Autodesk Inventor part; units mm, degrees
ref_plane "YZ Plane" through (0, 0, 0) normal (1, 0, 0) x (0, 1, 0)
ref_plane "XZ Plane" through (0, 0, 0) normal (0, 1, 0) x (-1, 0, 0)
ref_plane "XY Plane" through (0, 0, 0) normal (0, 0, 1) x (1, 0, 0)
sketch "Sketch1" plane through (0, 0, 0) normal (0, 1, 0) x (-1, 0, 0)
  arc A0 (-99.8914, -75.1446) -> (-99.8914, 75.1446) centre (0, 0) ccw
  line L0 (-65, 0) -> (-65, 55)
  line L1 (-65, 55) -> (-99.8914, 75.1446)
  line L2 (-65, 0) -> (-65, -55)
  line L3 (-65, -55) -> (-99.8914, -75.1446)
  dimension "d0" = 250
  dimension "d4" = 55
  dimension "d6" = 120
extrude "Extrusion1" add sketch "Sketch1" along normal blind 5
sketch "Sketch2" plane through (0, 5, 0) normal (0, 1, 0) x (1, 0, 0)
  line L0 (-70, 15) -> (15, 15)
  line L1 (15, 40) -> (-70, 40)
  arc A0 (15, 15) -> (15, 40) centre (15, 27.5) ccw
  arc A1 (-70, 40) -> (-70, 15) centre (-70, 27.5) ccw
  line L2 (65, -55) -> (65, 55)
  line L3 (-70, -15) -> (15, -15)
  line L4 (15, -40) -> (-70, -40)
  arc A2 (15, -40) -> (15, -15) centre (15, -27.5) ccw
  arc A3 (-70, -15) -> (-70, -40) centre (-70, -27.5) ccw
  point P0 (0, 0)
extrude "Extrusion2" cut sketch "Sketch2" against normal blind 10
sketch "Sketch3" plane through (0, 5, 0) normal (0, 1, 0) x (1, 0, 0)
  circle A0 centre (-105, 0) radius 4
  circle A1 centre (0, 105) radius 4.3333
  circle A2 centre (0, -105) radius 4.3461
  arc A3 (99.8914, 75.1446) -> (99.8914, -75.1446) centre (0, 0) ccw
  dimension "d25" = 8
  dimension "d26" = 105
  dimension "d27" = 105
  dimension "d28" = 105
extrude "Extrusion3" cut sketch "Sketch3" against normal blind 10
sketch "Sketch4" plane through (0, 5, 0) normal (0, 1, 0) x (1, 0, 0)
  circle A0 centre (-59.9853, -55) radius 2.5
  circle A1 centre (-29.9853, -55) radius 5
  circle A2 centre (0.0147, -55) radius 5
  line L0 (-104.2134, 0) -> (86.9491, 0)
  point P0 (0, 0)
  dimension "d31" = 5
  dimension "d32" = 10
  dimension "d33" = 10
  dimension "d34" = 55
  dimension "d35" = 55
  dimension "d36" = 55
  dimension "d37" = 30
  dimension "d38" = 30
extrude "Extrusion4" add sketch "Sketch4" along normal blind 10
fillet "Fillet2" radius 2 1 edges at (-62.4853, 15, 55)
chamfer "Chamfer1" distance 1.25 angle 45 1 edges at (-4.9853, 15, 55)
chamfer "Chamfer2" distance 1.25 angle 45 1 edges at (-34.9853, 15, 55)
sketch "Sketch5" plane through (0, 5, 0) normal (0, 1, 0) x (1, 0, 0)
  line L0 (-35.937, -60.9099) -> (-23.937, -60.9099)
  line L1 (-23.937, -60.9099) -> (-23.937, -48.9099)
  line L2 (-23.937, -48.9099) -> (-35.937, -48.9099)
  line L3 (-35.937, -48.9099) -> (-35.937, -60.9099)
  point P0 (0, 0)
  point P1 (-29.437, -54.7059)
  point P2 (-29.437, -54.7059)
  dimension "d50" = 12
  dimension "d51" = 12
  dimension "d52" = 6.5
  dimension "d53" = 5.796
extrude "Extrusion5" add sketch "Sketch5" along normal blind 0.05
sketch "Sketch6" plane through (0, 5, 0) normal (0, 1, 0) x (1, 0, 0)
  line L0 (-36.7143, -61.9407) -> (-23.1511, -61.9407) construction
  line L1 (-23.1511, -61.9407) -> (-23.1511, -65.2373) construction
  line L2 (-23.1511, -65.2373) -> (-36.7143, -65.2373) construction
  line L3 (-36.7143, -65.2373) -> (-36.7143, -61.9407) construction
  point P0 (0, 0)
properties part number "Top and middle round"
Design review of the part built by this model. Coordinates are the model's own, in mm. A direction names the side the tool comes from. Round coordinates to 2 decimals unless told otherwise and drop trailing zeros. Loops run counter-clockwise (first coordinate to the right, second up) from the corner with the lowest first, then second, coordinate; pieces in that order, holes last. Notation, with made-up numbers: (64, -30) - (102, -30) arc R17 ccw to (102, -17) - close; hole circle Ø11 at (16, 80). An arc over 180 degrees is marked (long way). One line per item, written item: value. Start each with the question number.
1) Consider section B-B on x = -79.5. Give the boundary of the cut face in (y, z), then the cut area to 3 significant figures.
2) Consider section D-D on z = 0. Give the boundary of the cut face in (x, y).
3) Consider section C-C on y = 8. Give the boundary of the cut face in (x, z).
4) Consider section A-A on z = -27.5. Give the boundary of the cut face in (x, y), then the cut area to 3 significant figures.
5) Draft analysis for pull direction Z (two halves, no side actions). For faces 4 (the cylindrical face through (-0.564, 2.535, -109.296)), 5 (the cylindrical face through (-124.924, 2.465, 4.368)), 6 (the flat face through (-11, 0, 2)), state which applies: +Z half, -Z half, draft (parallel to the pull), parting line (faces both ways), or undercut.
6) To check wall thickness, follow L1, parallel to Z at x = 0, y = 1.55; L2, parallel to X at y = 3.4, z = 0; L3, parallel to Z at x = -32, y = 2.75. State the ranges of each line that lie inside material, in increasing order. Write a range as from..to.
7) Insertion check: pin 1 Ø10 at (x, z) = (-7.5, 0.5) entering from +Y; pin 2 Ø11.5 at (x, z) = (0, -105) entering from -Y; pin 3 Ø4 at (x, y) = (-43, 3) entering from -Z; pin 4 Ø2.5 at (x, y) = (-32.5, 3.5) entering from +Z. Each pin has a flat end and moves straight along its axis. Give the tip position at first contact, or say it passes through.
8) For faces 1 (the cylindrical face through (-82.497, 2.535, 27.225)), 2 (the flat face through (82.2, 2.46, 64.93)), 3 (the cylindrical face through (-0.636, 9.314, 59.957)), list the 3-axis set-ups (+Z, -Z, +X, -X, +Y, -Y) from which the entire face can be reached by the end or side of a thin tool; tool diameter is ignored.
Reported:
1. outline: (0, -96.46) - (5, -96.46) - (5, -35.62) - (0, -35.62) - close; (0, -19.38) - (5, -19.38) - (5, 19.38) - (0, 19.38) - close; (0, 35.62) - (5, 35.62) - (5, 96.46) - (0, 96.46) - close
1. area: 802 mm^2
2. outline: (-125, 0) - (-109, 0) - (-109, 5) - (-125, 5) - close; (-101, 0) - (65, 0) - (65, 5) - (-101, 5) - close
3. outline: circle Ø5 at (-59.99, 55); circle Ø10 at (-29.99, 55); circle Ø10 at (0.01, 55)
4. outline: (-121.94, 0) - (-82.5, 0) - (-82.5, 5) - (-121.94, 5) - close; (27.5, 0) - (65, 0) - (65, 5) - (27.5, 5) - close
4. area: 385 mm^2
5. face 4: undercut
5. face 5: parting line
5. face 6: draft
6. L1: z = -125..-109.33, -100.67..-40, -15..15, 40..100.65, 109.35..125
6. L2: x = -125..-109, -101..65
6. L3: z = -120.83..-40, -15..15, 40..120.83
7. pin 1: stops at y = 5
7. pin 2: stops at y = 0
7. pin 3: stops at z = -118.08
7. pin 4: stops at z = 121.03
8. face 1: +Y, -Y
8. face 2: +X, +Y, -Y
8. face 3: +Y
